Source: CAD feature listing. Evaluate the final solid. Frame: model axes, mm. Face numbers are marked on the shaded views. A direction names the side the tool comes from. Give positions to 0.01 mm unless a question says otherwise; leave off trailing zeros. Order: outer loops, then holes, each group sorted by start corner. A loop starts at its lowest first (then second) coordinate and runs counter-clockwise, first axis right, second up.
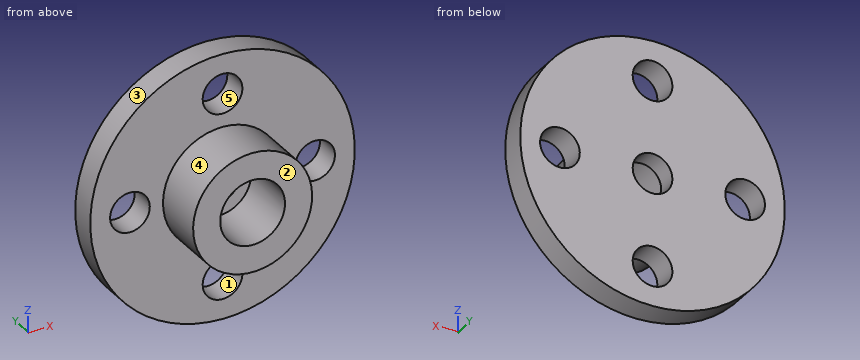
from build123d import *

# Parameters (mm, degrees)
SKETCH_1_R               = 10
SKETCH_1_R_2             = 1.5
EXTRUDE_1_DEPTH          = 2
SKETCH_2_R               = 4.5
EXTRUDE_2_DEPTH          = 4
CUT_EXTRUDE_1_DEPTH      = 15.696938457
CUT_EXTRUDE_1_DEPTH_BACK = 15.696938457
SKETCH_3_R               = 1.5
CUT_EXTRUDE_START        = -4
SKETCH_4_R               = 2.45
CUT_EXTRUDE_2_DEPTH      = 4.5


with BuildPart() as part:
    # 草图1 → 凸台-拉伸1 (new body)
    with BuildSketch(Plane(origin=(0, 0, 0), x_dir=(1, 0, 0), z_dir=(0, 1, 0))):
        with Locations(Location((0, 0, 0), (0, 0, 270))):
            Circle(SKETCH_1_R)
        with Locations(Location((0, 7, 0), (0, 0, 270))):
            Circle(SKETCH_1_R_2, mode=Mode.SUBTRACT)
        with Locations(Location((7, 0, 0), (0, 0, 270))):
            Circle(SKETCH_1_R_2, mode=Mode.SUBTRACT)
        with Locations(Location((0, -7, 0), (0, 0, 270))):
            Circle(SKETCH_1_R_2, mode=Mode.SUBTRACT)
        with Locations(Location((-7, 0, 0), (0, 0, 270))):
            Circle(SKETCH_1_R_2, mode=Mode.SUBTRACT)
    extrude(amount=EXTRUDE_1_DEPTH)

    # 草图2 → 凸台-拉伸2 (add)
    with BuildSketch(Plane(origin=(0, 0, 0), x_dir=(1, 0, 0), z_dir=(0, 1, 0))):
        with Locations(Location((0, 0, 0), (0, 0, 270))):
            Circle(SKETCH_2_R)
    extrude(amount=-EXTRUDE_2_DEPTH)

    # 草图3 → 切除-拉伸1 (cut, two sides: drawn at the far end of the back side and taken through both)
    with BuildSketch(Plane(origin=(0, 0, 0), x_dir=(1, 0, 0), z_dir=(0, 1, 0)).offset(-CUT_EXTRUDE_1_DEPTH_BACK)):
        with Locations(Location((0, 0, 0), (0, 0, 270))):
            Circle(SKETCH_3_R)
    extrude(amount=CUT_EXTRUDE_1_DEPTH + CUT_EXTRUDE_1_DEPTH_BACK, mode=Mode.SUBTRACT)

    # 草图4 → 切除-拉伸2 (cut)
    with BuildSketch(Plane(origin=(0, 0, 0), x_dir=(1, 0, 0), z_dir=(0, 1, 0)).offset(CUT_EXTRUDE_START)):
        with Locations(Location((0, 0, 0), (0, 0, 270))):
            Circle(SKETCH_4_R)
    extrude(amount=CUT_EXTRUDE_2_DEPTH, mode=Mode.SUBTRACT)


solid = part.part
(1) Section A-A, the plane z = 0. Return loops of the section in (x, y).
(2) Pin query (flat end, axial travel): pin 1 Ø4.5 at (x, z) = (0, 0) entering from -Y; pin 2 Ø2.5 at (x, z) = (0, 0) entering from -Y; pin 3 Ø1 at (x, y) = (5, 0) entering from +Z; pin 4 Ø2 at (x, z) = (7.5, 5.5) entering from -Y. Return the tip coordinate at first contact, or that it passes through.
(3) Section C-C, the plane z = -7. Return loops of the section in (x, y), plus the area to 3 significant figures.
(4) Line query: line 1 along X through (y, z) = (1.05, 0); line 2 along Y through (x, z) = (-2.5, 5.75); line 3 along Z through (x, y) = (6.75, 1). Output: solid intervals per line, ascending.
(5) Access query for the marked faces 4 and 5. Directions: +Z, -Z, +X, -X, +Y, -Y. A direction counts if a zero-diameter tool reaches every point of the face in a straight line with its end or side. Return the directions, or none.
(6) Section D-D, the plane x = -8. Return loops of the section in (y, z), plus the area to 3 significant figures.
(7) Draft query along X for the marked faces 1, 2 and 3. Return one class per face: +X half, -X half, draft (parallel to the pull), parting line (faces both ways), or undercut.
(8) Section B-B, the plane x = 0. Return loops of the section in (y, z), plus the area to 4 significant figures.
Checks:
1. outline: (-10, 0) - (-8.5, 0) - (-8.5, 2) - (-10, 2) - close; (-5.5, 0) - (-4.5, 0) - (-4.5, -4) - (-2.45, -4) - (-2.45, 0.5) - (-1.5, 0.5) - (-1.5, 2) - (-5.5, 2) - close; (1.5, 0.5) - (2.45, 0.5) - (2.45, -4) - (4.5, -4) - (4.5, 0) - (5.5, 0) - (5.5, 2) - (1.5, 2) - close; (8.5, 0) - (10, 0) - (10, 2) - (8.5, 2) - close
2. pin 1: stops at y = 0.5
2. pin 2: passes through
2. pin 3: stops at z = 8.93
2. pin 4: stops at y = 0
3. outline: (-7.14, 0) - (-1.5, 0) - (-1.5, 2) - (-7.14, 2) - close; (1.5, 0) - (7.14, 0) - (7.14, 2) - (1.5, 2) - close
3. area: 22.6 mm2
4. line 1: x = -10 to -8.5, -5.5 to -1.5, 1.5 to 5.5, 8.5 to 10
4. line 2: y = 0 to 2
4. line 3: z = -7.38 to -1.48, 1.48 to 7.38
5. face 4: -Y
5. face 5: +Y, -Y
6. outline: (0, -6) - (2, -6) - (2, -1.12) - (0, -1.12) - close; (0, 1.12) - (2, 1.12) - (2, 6) - (0, 6) - close
6. area: 19.5 mm2
7. face 1: undercut
7. face 2: draft
7. face 3: parting line
8. outline: (-4, -4.5) - (0, -4.5) - (0, -5.5) - (2, -5.5) - (2, -1.5) - (0.5, -1.5) - (0.5, -2.45) - (-4, -2.45) - close; (-4, 2.45) - (0.5, 2.45) - (0.5, 1.5) - (2, 1.5) - (2, 5.5) - (0, 5.5) - (0, 4.5) - (-4, 4.5) - close; (0, -10) - (2, -10) - (2, -8.5) - (0, -8.5) - close; (0, 8.5) - (2, 8.5) - (2, 10) - (0, 10) - close
8. area: 37.45 mm2
